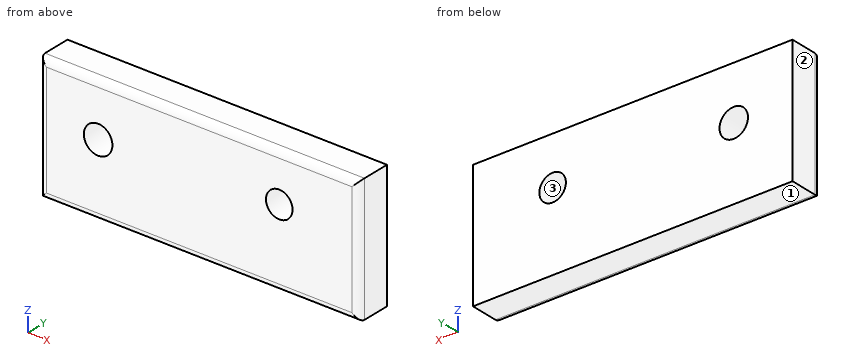
```python
from build123d import *

# Parameters (mm, degrees)
F0_W     = 233.076439
F0_H     = 91.861807
F1_DEPTH = 25.4
F2_R     = 5.08
F3_R     = 10.397346
F3_R_2   = 9.68524
F4_DEPTH = 25.4


with BuildPart() as f1:
    # F0 (on Front) → F1 (new body)
    with BuildSketch(Plane.XZ):
        with Locations((1.484566, 7.702914)):
            Rectangle(F0_W, F0_H)
    extrude(amount=F1_DEPTH)

    # F2
    f2_edges = [f1.edges().sort_by_distance(p)[0] for p in [
        (1.484565, -25.4, 53.633817),
        (-115.053654, -25.4, 7.702913),
        (1.484565, -25.4, -38.22799),
        (118.022785, -25.4, 7.702913),
    ]]
    fillet(f2_edges, radius=F2_R)

    # F3 (on face) → F4 (cut)
    with BuildSketch(Plane.XZ.offset(25.4)):
        with Locations((-72.182253, 14.576591)):
            Circle(F3_R)
        with Locations((59.943877, 18.573165)):
            Circle(F3_R_2)
    extrude(amount=-F4_DEPTH, mode=Mode.SUBTRACT)


solid = f1.part
```
Geometry check sheet. Reference: the model listing, model coordinates, mm. Face numbers are marked on the shaded views. Coordinates: 2 decimals unless noted, no trailing zeros. Order: outer loops, then holes, each group sorted by start corner. A loop starts at its lowest first (then second) coordinate and runs counter-clockwise, first axis right, second up. Notation, with made-up numbers: M -3.5,2 L 5.5,2 A26 ccw 5.5,20 Z; hole C 45.25,2 d6. An arc over 180 degrees is marked long. Answer as a JSON object with one key per item and string values.
Q1. Release check for a two-part mould opening along X. For the marked faces 1, 2 and 3 record: released by +X, released by -X, zero draft, split by the parting line, or undercut.
Results are:
{"face 1": "zero draft", "face 2": "released by -X", "face 3": "undercut"}
Q2. Cross-section at C-C on x = 60. Record the cut outline in (y, z).
Results are:
{"outline": "M -25.4,-33.15 A5.08 ccw -20.32,-38.23 L 0,-38.23 L 0,8.89 L -25.4,8.89 Z; M -25.4,28.26 L 0,28.26 L 0,53.63 L -20.32,53.63 A5.08 ccw -25.4,48.55 Z"}
Q3. Cross-section at B-B on x = -69. Record the cut outline in (y, z), and give its area (3 significant figures).
Results are:
{"outline": "M -25.4,-33.15 A5.08 ccw -20.32,-38.23 L 0,-38.23 L 0,4.68 L -25.4,4.68 Z; M -25.4,24.47 L 0,24.47 L 0,53.63 L -20.32,53.63 A5.08 ccw -25.4,48.55 Z", "area": "1,820 mm²"}
Q4. Depth check by flat-ended pin: pin 1 Ø1 at (x, y) = (80, -22) entering from -Z. Enter the tip coordinate at first touch or a pass-through.
Results are:
{"pin 1": "stops at z = -38.09"}
Q5. Cross-section at A-A on y = -3.75. Record the cut outline in (x, z), and give its area (3 significant figures).
Results are:
{"outline": "M -115.05,-38.23 L 118.02,-38.23 L 118.02,53.63 L -115.05,53.63 Z; hole C -72.18,14.58 d20.79; hole C 59.94,18.57 d19.37", "area": "20,800 mm²"}
Q6. Scan lines: line 1 (X direction, y = -22.5, z = 12); line 2 (X direction, y = -5.75, z = 14); line 3 (Z direction, x = 58, y = -2.5) (3 decimals). Record each from-to range of solid material in increasing order.
Results are:
{"line 1": "x = -114.56 to -82.26, -62.11 to 52.83, 67.06 to 117.53", "line 2": "x = -115.05 to -82.56, -61.8 to 51.41, 68.48 to 118.02", "line 3": "z = -38.228 to 9.085, 28.061 to 53.634"}
